from build123d import *

# Parameters (mm, degrees)
F1_DEPTH = 25.4
F2_R     = 3.175
F3_DEPTH = 25.4
F4_R     = 3.175
F5_DEPTH = 28.448


with BuildPart() as f1:
    # F0 (on Top) → F1 (new body)
    with BuildSketch(Plane.XY):
        Polygon((0, 28.448), (0, 0), (66.548, 0), (66.548, 28.448), (28.448, 28.448), (28.448, 6.35), (25.4, 6.35), (25.4, 28.448), align=None)
    extrude(amount=F1_DEPTH)

    # F2 (on face) → F3 (cut)
    with BuildSketch(Plane.XY.offset(25.4)):
        with Locations((6.35, 6.35)):
            Circle(F2_R)
        with Locations((60.198, 6.35)):
            Circle(F2_R)
        with Locations((60.198, 22.098)):
            Circle(F2_R)
        with Locations((6.35, 22.098)):
            Circle(F2_R)
    extrude(amount=-F3_DEPTH, mode=Mode.SUBTRACT)

    # F4 (on face) → F5 (cut, through all)
    with BuildSketch(Plane(origin=(0, 28.448, 0), x_dir=(-1, 0, 0), z_dir=(0, 1, 0))):
        with Locations((-34.798, 6.35)):
            Circle(F4_R)
        with Locations((-34.798, 19.05)):
            Circle(F4_R)
    extrude(amount=-F5_DEPTH, mode=Mode.SUBTRACT)


solid = f1.part
CAD build for the part. Positions are in the model's coordinates, mm. A direction names the side the tool comes from. Round coordinates to 2 decimals unless told otherwise and drop trailing zeros. Loops run counter-clockwise (first coordinate to the right, second up) from the corner with the lowest first, then second, coordinate; pieces in that order, holes last.
(1) Which spindle directions (+Z, -Z, +X, -X, +Y, -Y) get a long thin tool onto all of the face, cutting with end or side? Do faces 4 (the flat face through (25.4, 17, 13)), 5 (the cylindrical face through (59.5, 19, 12.9)). Say none if no direction does.
(2) Wall check: line 1 along Z through (x, y) = (35, 25.5); line 2 along Y through (x, z) = (60, 18.25); line 3 along X through (y, z) = (11, 23.5). Give the ranges that are in metal, low to high.
(3) Cut at A-A (y = 12.75). Give the cut face in (x, z) (3 decimals).
(4) Cut at C-C (z = 5). Give the cut face in (x, y) (3 decimals), plus the area to 3 significant figures.
(5) Cut at D-D (y = 22.75). Give the cut face in (x, z) (3 decimals), plus the area to 3 significant figures.
(6) Drop flat-ended pins along their axis: pin 1 (0.9 mm diameter, centred on x = 26.5, z = 6.5, fed in from +Y); pin 2 (4 mm diameter, centred on x = 34.798, z = 6.35, fed in from +Y) (3 decimals); pin 3 (8.5 mm diameter, centred on x = 60.198, y = 6.35, fed in from -Z). Give the stop position or say it passes through.
(7) Cut at B-B (x = 6.35). Give the cut face in (y, z) (3 decimals), plus the area to 3 significant figures.
(8) Two-plate mould, pull along Y, no slides. Class faces 1 (the cylindrical face through (4.01, 8.496, 12.878)), 2 (the flat face through (33, 0, 13)), 3 (the flat face through (66.548, 14, 13)): +Y half, -Y half, draft (parallel to the pull), parting line (faces both ways), or undercut.
Findings below:
1. face 4: +Z, -Z, +Y
1. face 5: +Z, -Z
2. line 1: z = 0 to 3.18, 9.52 to 15.88, 22.22 to 25.4
2. line 2: y = 0 to 3.18, 9.52 to 18.93, 25.27 to 28.45
2. line 3: x = 0 to 25.4, 28.45 to 66.55
3. outline: (0, 0) - (25.4, 0) - (25.4, 25.4) - (0, 25.4) - close; (28.448, 0) - (66.548, 0) - (66.548, 25.4) - (28.448, 25.4) - close; hole circle Ø6.35 at (34.798, 6.35); hole circle Ø6.35 at (34.798, 19.05)
4. outline: (0, 0) - (31.924, 0) - (31.924, 28.448) - (28.448, 28.448) - (28.448, 6.35) - (25.4, 6.35) - (25.4, 28.448) - (0, 28.448) - close; (37.672, 0) - (66.548, 0) - (66.548, 28.448) - (37.672, 28.448) - close; hole circle Ø6.35 at (6.35, 6.35); hole circle Ø6.35 at (6.35, 22.098); hole circle Ø6.35 at (60.198, 6.35); hole circle Ø6.35 at (60.198, 22.098)
4. area: 1,540 mm2
5. outline: (0, 0) - (3.243, 0) - (3.243, 25.4) - (0, 25.4) - close; (9.457, 0) - (25.4, 0) - (25.4, 25.4) - (9.457, 25.4) - close; (28.448, 0) - (57.091, 0) - (57.091, 25.4) - (28.448, 25.4) - close; (63.305, 0) - (66.548, 0) - (66.548, 25.4) - (63.305, 25.4) - close; hole circle Ø6.35 at (34.798, 6.35); hole circle Ø6.35 at (34.798, 19.05)
5. area: 1,230 mm2
6. pin 1: stops at y = 6.35
6. pin 2: passes through
6. pin 3: stops at z = 0
7. outline: (0, 0) - (3.175, 0) - (3.175, 25.4) - (0, 25.4) - close; (9.525, 0) - (18.923, 0) - (18.923, 25.4) - (9.525, 25.4) - close; (25.273, 0) - (28.448, 0) - (28.448, 25.4) - (25.273, 25.4) - close
7. area: 400 mm2
8. face 1: undercut
8. face 2: -Y half
8. face 3: draft
